Here's how the part is built. I have some questions about the finished solid (model axes, mm). Face numbers are marked on the shaded views. A direction names the side the tool comes from. Round coordinates to 2 decimals unless told otherwise and drop trailing zeros. Order: outer loops, then holes, each group sorted by start corner. A loop starts at its lowest first (then second) coordinate and runs counter-clockwise, first axis right, second up. Notation, with made-up numbers: (31, 20.25) -> (37, 20.25) arc R14 ccw to (37, 36.25) -> close; hole circle Ø9 at (-7, 62). An arc over 180 degrees is marked (long way). Answer in a Markdown table with one row per item.
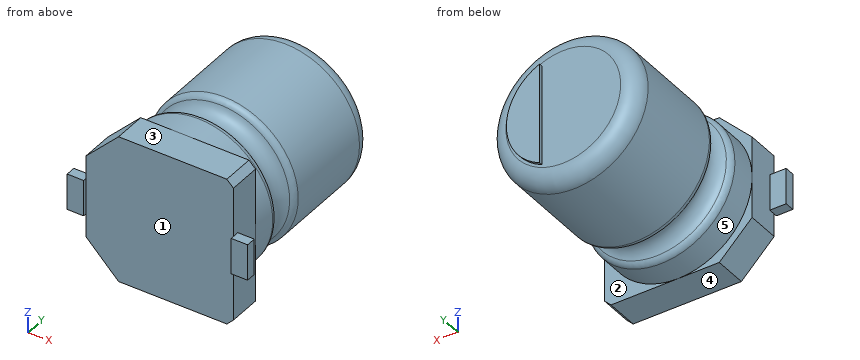
Autodesk Inventor part; units mm, degrees
ref_plane "YZ Plane" through (0, 0, 0) normal (1, 0, 0) x (0, 1, 0)
ref_plane "XZ Plane" through (0, 0, 0) normal (0, 1, 0) x (-1, 0, 0)
ref_plane "XY Plane" through (0, 0, 0) normal (0, 0, 1) x (1, 0, 0)
sketch "Sketch1" plane through (0, 0, 0) normal (0, 1, 0) x (-1, 0, 0)
  line L0 (2.25, 2.25) -> (-2.25, 2.25)
  line L1 (-2.25, 2.25) -> (-2.25, -2.25)
  line L2 (-2.25, -2.25) -> (2.25, -2.25)
  line L3 (2.25, -2.25) -> (2.25, 2.25)
  line L4 (2.25, 1.25) -> (1.25, 2.25)
  line L5 (2.25, -1.25) -> (1.25, -2.25)
  point P0 (0, 0)
  dimension "d0" = 4.5
  dimension "d1" = 4.5
  dimension "d2" = 2.25
  dimension "d3" = 2.25
  dimension "d4" = 45
  dimension "d5" = 45
  dimension "d6" = 1
  dimension "d7" = 1
extrude "Extrusion1" add sketch "Sketch1" along normal blind 1 contours L4 L3 L5 L2 L1 L0
chamfer "Chamfer1" distance 0.2 angle 45 2 edges at (2.25, 0.5, 2.25) (2.25, 0.5, -2.25)
sketch "Sketch2" plane through (0, 1, 0) normal (0, 1, 0) x (1, 0, 0)
  circle A0 centre (0, 0) radius 2.25
  dimension "d13" = 4.5
extrude "Extrusion2" add sketch "Sketch2" along normal blind 5.2
sketch "Sketch3" plane through (0, 0, 0) normal (0, -1, 0) x (1, 0, 0)
  line L0 (-2.25, 0.55) -> (-2.25, -0.55)
  line L1 (-2.75, -0.55) -> (-2.75, 0.55)
  line L2 (-2.75, 0.55) -> (-2.25, 0.55)
  line L3 (-2.75, -0.55) -> (-2.25, -0.55)
  point P0 (0, 0)
  dimension "d16" = 1.1
  dimension "d18" = 2.25
  dimension "d33" = 2.75
extrude "Extrusion3" add sketch "Sketch3" along normal blind 0.1 and the other way blind 0.2
mirror "Mirror1" about plane through (0, 0, 0) normal (1, 0, 0) of "Extrusion3"
fillet "Fillet1" radius 0.5 1 edges at (-2.25, 6.2, 0)
sketch "Sketch4" plane through (0, 6.2, 0) normal (0, 1, 0) x (1, 0, 0)
  circle A0 centre (0, 0) radius 6.25
  circle A1 centre (0, 0) radius 2.25
  line L0 (3.2451, -4.6893) -> (3.2427, 4.6909)
  arc A2 (3.2451, -4.6893) -> (3.2427, 4.6909) centre (0, 0) ccw
  arc A3 (0.6558, -1.5332) -> (0.6558, 1.5332) centre (0, 0) ccw
  line L1 (0.6558, -1.5332) -> (0.6558, 1.5332)
extrude "Extrusion5" add sketch "Sketch4" along normal blind 0.1 contours L1 A3
sketch "Sketch5" plane through (0, 0, 0) normal (0, 0, 1) x (1, 0, 0)
  line L0 (2.25, 1) -> (2.25, 5.7)
  line L1 (0, -1.3032) -> (0, 7.8193)
  circle A0 centre (2.25, 2.3529) radius 0.4103
  point P0 (0, 0)
revolve "Revolution1" cut sketch "Sketch5" angle 360 about axis through (0, -10, 0) along (0, 1, 0)
fillet "Fillet4" radius 0.2 2 edges at (-2.25, 1.9426, 0) (-2.25, 2.7632, 0)
properties part number "SMTElectro4x4x6_5"
1. We'd pull the mould along Y, two halves only. Please class the marked faces 1, 2 and 3: released by +Y, released by -Y, zero draft, split by the parting line, or undercut.
Numbers:
| item | result |
|---|---|
| face 1 | released by -Y |
| face 2 | released by +Y |
| face 3 | zero draft |
2. Suppose I cut it at C-C on y = 2.25. Write out the boundary of the cut face in (x, z), then the cut area to 3 significant figures.
Numbers:
| item | result |
|---|---|
| outline | circle Ø3.71 at (0, 0) |
| area | 10.8 mm2 |
3. For pin 1 Ø1.8 at (x, z) = (1.5, -1.5) entering from +Y; pin 2 Ø1.8 at (x, z) = (-1, -1.5) entering from +Y; pin 3 Ø1.5 at (x, z) = (1.5, 1) entering from -Y, each with a flat end and sliding along its axis, tell me the tip position at first contact or that it passes through.
Numbers:
| item | result |
|---|---|
| pin 1 | stops at y = 6.3 |
| pin 2 | stops at y = 6.2 |
| pin 3 | stops at y = 0 |
4. For the marked faces 4 and 5, which set-ups out of +Z, -Z, +X, -X, +Y, -Y let a thin tool reach every point of the face, with its end or its side?
Numbers:
| item | result |
|---|---|
| face 4 | -Z, +X, -X, +Y, -Y |
| face 5 | +Y |
5. Suppose I cut it at B-B on y = 4. Write out the boundary of the cut face in (x, z), then the cut area to 3 significant figures.
Numbers:
| item | result |
|---|---|
| outline | circle Ø4.5 at (0, 0) |
| area | 15.9 mm2 |
6. Please list where these lines run through material, in increasing order: line 1 along Y through (x, z) = (-1.8, 1.1); line 2 along Y through (x, z) = (-0.5, 0.4); line 3 along X through (y, z) = (0.5, 0).
Numbers:
| item | result |
|---|---|
| line 1 | y = 0 to 1.97, 2.74 to 6.05 |
| line 2 | y = 0 to 6.2 |
| line 3 | x = -2.25 to 2.25 |
7. Suppose I cut it at A-A on y = 0.5. Write out the boundary of the cut face in (x, z).
Numbers:
| item | result |
|---|---|
| outline | (-2.25, -1.25) -> (-1.25, -2.25) -> (2.05, -2.25) -> (2.25, -2.05) -> (2.25, 2.05) -> (2.05, 2.25) -> (-1.25, 2.25) -> (-2.25, 1.25) -> close |
